Read the model definition and answer for the solid it produces. Units are mm, in the model's axes. Face numbers are marked on the shaded views. A direction names the side the tool comes from. Give positions to 0.01 mm unless a question says otherwise; leave off trailing zeros. Write each loop counter-clockwise with the first axis right and the second up, starting at its lowest first coordinate (ties: lowest second). Pieces come first, ordered by that corner, then holes. Notation, with made-up numbers: (3, 10) -> (38, 10) arc R29 cw to (38, 31) -> close; hole circle Ø8 at (69, 30). An arc over 180 degrees is marked (long way). Write item = value, one per line.
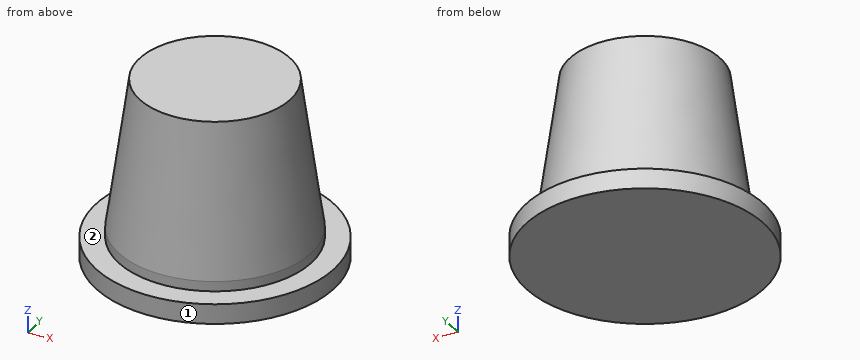
Autodesk Inventor part; units mm, degrees
ref_plane "YZ Plane" through (0, 0, 0) normal (1, 0, 0) x (0, 1, 0)
ref_plane "XZ Plane" through (0, 0, 0) normal (0, 1, 0) x (-1, 0, 0)
ref_plane "XY Plane" through (0, 0, 0) normal (0, 0, 1) x (1, 0, 0)
sketch "Sketch1" plane through (0, 0, 0) normal (0, 0, 1) x (1, 0, 0)
  arc A0 (-34.8899, -33.6307) -> (-34.8899, -38.7172) centre (-36.3549, -36.1739) ccw
  circle A1 centre (-36.3549, -36.1739) radius 9.6697
  point P0 (0, 0)
extrude "Extrusion1" add sketch "Sketch1" along normal blind 18
chamfer "Chamfer2" distance 15 angle 8 1 edges at (-46.0245, -36.1739, 18) measured on face at (-26.7165, -36.952, 12)
ref_plane "Work Plane1" through (0, 0, 0) normal (0, 0, 1) x (1, 0, 0)
sketch "Sketch2" plane through (0, 0, 0) normal (0, 0, 1) x (1, 0, 0)
  circle A0 centre (-36.3549, -36.1739) radius 7.5616
  circle A1 centre (-36.3549, -36.1739) radius 11.9385
  point P0 (0, 0)
extrude "Extrusion2" add sketch "Sketch2" along normal blind 2
properties part number "Knob"
(1) The part is cut by section C-C on z = 13.25. Determine the outline of the cut face in (x, y).
Checks:
outline = circle Ø16.46 at (-36.35, -36.17)
(2) A tool of negligible diameter and unlimited length cuts with its end or side. For the marked faces 1 and 2, from which of +Z, -Z, +X, -X, +Y, -Y can it reach the whole face along a straight path? Write none if from no direction.
Checks:
face_1 = +Z, -Z
face_2 = +Z
(3) Given P1, Ø5, axis at x = -45.5, y = -28, coming from the +Z side; P2, Ø2, axis at y = -44.5, z = 4.5, coming from the +X side; P3, Ø4, axis at x = -38.5, z = 4.5, coming from the +Y side, each flat-ended and moving along its own axis, determine where each tip first touches the part or whether it passes through.
Checks:
P1 = 2
P2 = -30.35
P3 = -26.54
(4) The part is cut by section B-B on z = 10. Determine the outline of the cut face in (x, y), plus the area to 3 significant figures.
Checks:
outline = circle Ø17.37 at (-36.35, -36.17)
area = 237 mm²
(5) Consider L1, parallel to Z at x = -27.5, y = -29.5; L2, parallel to Y at x = -33.5, z = 15; L3, parallel to Y at x = -29.5, z = 16.5. Determine where each line is inside the solid, lowest interval first.
Checks:
L1 = 0 to 2
L2 = -43.63 to -28.72
L3 = -39.84 to -32.51
(6) The part is cut by section A-A on y = -26. Determine the outline of the cut face in (x, z), plus the area to 3 significant figures.
Checks:
outline = (-42.6, 0) -> (-30.11, 0) -> (-30.11, 2) -> (-42.6, 2) -> close
area = 25.0 mm²
